Source: CAD feature listing. Evaluate the final solid. Frame: model axes, mm. A direction names the side the tool comes from. Give positions to 0.01 mm unless a question says otherwise; leave off trailing zeros. Loops run counter-clockwise (first coordinate to the right, second up) from the corner with the lowest first, then second, coordinate; pieces in that order, holes last. Notation, with made-up numbers: M 47.5,-19.5 L 93.5,-19.5 A19 ccw 93.5,-5.5 Z; hole C 1,-28.75 d5. An arc over 180 degrees is marked long. Put each result on its own line as item: value. Start each with the question number.
```python
from build123d import *

# Parameters (mm, degrees)
SKETCH1_R           = 6.35
BOSS_EXTRUDE1_DEPTH = 19.05


with BuildPart() as part:
    # Sketch1 → Boss-Extrude1 (new body)
    with BuildSketch(Plane(origin=(0, 0, 0), x_dir=(1, 0, 0), z_dir=(0, 1, 0))):
        Polygon((0, 0), (190.5, 0), (190.5, 12.7), (165.1, 12.7), (83.222475072, 114.3), (60.362475072, 114.3), (60.362475072, 47.594615045), (31.75, 12.7), (0, 12.7), align=None)
        with Locations(Location((71.413185557, 86.36, 0), (0, 0, 90))):
            Circle(SKETCH1_R, mode=Mode.SUBTRACT)
        with Locations(Location((71.413185557, 50.8, 0), (0, 0, 90))):
            Circle(SKETCH1_R, mode=Mode.SUBTRACT)
        Polygon((81.72578072, 96.52), (81.72578072, 12.7), (147.76578072, 12.7), align=None, mode=Mode.SUBTRACT)
    extrude(amount=BOSS_EXTRUDE1_DEPTH)


solid = part.part
```
1. Section D-D, the plane z = -39.5. Output: boundary loops of the cut face in (x, y), plus the area to 3 significant figures.
2. Ray query, line 1 (X direction, y = 7.5, z = -50.8); line 2 (Z direction, x = 126, y = 5.25); line 3 (X direction, y = 8.75, z = -17.5). Return the intervals inside material, ascending.
3. Contact query for flat-ended pins moving along their axis: pin 1 (9.5 mm diameter, centred on x = 14, y = 6.5, fed in from -Z); pin 2 (5.5 mm diameter, centred on y = 12, z = -77.5, fed in from -X); pin 3 (4 mm diameter, centred on y = 2.5, z = -59, fed in from +X). Output: stop coordinate, or through.
4. Section B-B, the plane z = -86.36. Output: boundary loops of the cut face in (x, y).
5. Set-up query: faces 1 (the face through (60.362, 9, -81)), 2 (the face through (190.5, 9, -6)), 3 (the face through (178, 9, -12.7)), 4 (the face through (114, 9, -12.7)), 5 (the face through (94, 9, 0)). Return all of +Z, -Z, +X, -X, +Y, -Y with unobstructed straight access to the full face (end or side cutting, diameter ignored); none if empty.
6. Pull-direction query (X, two-part tool) for faces 6 (the face through (0, 9, -6)), 7 (the face through (16, 9, -12.7)), 8 (the face through (71.134, 9.392, -80.016)); classes: released by +X, released by -X, zero draft, split by the parting line, or undercut.
7. Section A-A, the plane x = 125. Output: boundary loops of the cut face in (y, z), plus the area to 3 significant figures.
8. Section C-C, the plane y = 8.5. Output: boundary loops of the cut face in (x, z).
Results found:
1. outline: M 53.73,0 L 81.73,0 L 81.73,19.05 L 53.73,19.05 Z; M 126.65,0 L 143.5,0 L 143.5,19.05 L 126.65,19.05 Z
1. area: 854 mm²
2. line 1: 60.36 to 65.06, 77.76 to 81.73, 117.75 to 134.4
2. line 2: -61.22 to -40.33, -12.7 to 0
2. line 3: 35.69 to 81.73, 143.98 to 161.23
3. pin 1: z = -12.7
3. pin 2: x = 60.36
3. pin 3: x = 129.4
4. outline: M 60.36,0 L 65.06,0 L 65.06,19.05 L 60.36,19.05 Z; M 77.76,0 L 81.73,0 L 81.73,19.05 L 77.76,19.05 Z; M 89.73,0 L 105.74,0 L 105.74,19.05 L 89.73,19.05 Z
5. face 1: -Z, -X, +Y, -Y
5. face 2: +Z, -Z, +X, +Y, -Y
5. face 3: -Z, +X, +Y, -Y
5. face 4: +Y, -Y
5. face 5: +Z, +X, -X, +Y, -Y
6. face 6: released by -X
6. face 7: zero draft
6. face 8: undercut
7. outline: M 0,-62.46 L 19.05,-62.46 L 19.05,-41.6 L 0,-41.6 Z; M 0,-12.7 L 19.05,-12.7 L 19.05,0 L 0,0 Z
7. area: 639 mm²
8. outline: M 0,-12.7 L 31.75,-12.7 L 60.36,-47.59 L 60.36,-114.3 L 83.22,-114.3 L 165.1,-12.7 L 190.5,-12.7 L 190.5,0 L 0,0 Z; hole C 71.41,-86.36 d12.7; hole C 71.41,-50.8 d12.7; hole M 81.73,-96.52 L 147.77,-12.7 L 81.73,-12.7 Z
